Geometry check sheet. Reference: the model listing, model coordinates, mm. Face numbers are marked on the shaded views. Give positions to 0.01 mm unless a question says otherwise; leave off trailing zeros. Write each loop counter-clockwise with the first axis right and the second up, starting at its lowest first coordinate (ties: lowest second). Pieces come first, ordered by that corner, then holes. Notation, with made-up numbers: (82.5, 85) - (94.5, 85) arc R14 cw to (94.5, 93) - close; hole circle Ø10 at (3.5, 63). An arc over 180 degrees is marked (long way). One line per question, with ' | ' between items. Start each with the question number.
Q1. Gauge pin test, flat ends, axial feed: P1, Ø1, axis at x = 6, y = 3, coming from the -Z side; P2, Ø1.5, axis at y = 3, z = -3.5, coming from the -X side; P3, Ø5, axis at x = 60, z = 0, coming from the +Y side. Record the tip position at first contact, or that the pin passes through.
Q2. Thickness scan on L1, parallel to X at y = 2.55, z = -1.25; L2, parallel to X at y = 4.05, z = -1.5; L3, parallel to Z at x = -2.5, y = 4.15. Record the ranges inside material, lowest first. Write a range as [from, to].
Q3. Section check A-A on y = 2.7. Record the boundary of the cut face in (x, z), and give its area (3 significant figures).
Q4. Section check C-C on z = -9. Record the boundary of the cut face in (x, y), and give its area (3 significant figures).
Q5. Release check for a two-part mould opening along Z. For the marked faces 1, 2, 3 and 4 record: +Z half, -Z half, draft (parallel to the pull), parting line (faces both ways), or undercut.
Q6. Section check B-B on x = 31.5. Record the boundary of the cut face in (y, z).
```python
from build123d import *

# Parameters (mm, degrees)
SKETCH_1_R      = 12.5
SKETCH_1_R_2    = 8
SKETCH_1_R_3    = 3.05
EXTRUDE_1_DEPTH = 5


with BuildPart() as part:
    # 草图1 → 凸台-拉伸1 (new body)
    # profile 1 of 3: a face of its own
    with BuildSketch(Plane(origin=(0, 0, 0), x_dir=(1, 0, 0), z_dir=(0, 1, 0))):
        with BuildLine():
            ThreePointArc((12.5, 0), (9.164298937, -8.500919068), (0.9375, -12.464794172))
            Line((0.9375, -12.464794172), (60.6, -7.97746827))
            ThreePointArc((60.6, -7.97746827), (52, 0), (60.6, 7.97746827))
            Line((60.6, 7.97746827), (0.9375, 12.464794172))
            ThreePointArc((0.9375, 12.464794172), (9.164298937, 8.500919068), (12.5, 0))
        make_face()
    # profile 2 of 3: a face of its own
    with BuildSketch(Plane(origin=(0, 0, 0), x_dir=(1, 0, 0), z_dir=(0, 1, 0))):
        Circle(SKETCH_1_R)
        Polygon((0, -7.071067812), (7.071067812, 0), (0, 7.071067812), (-7.071067812, 0), align=None, mode=Mode.SUBTRACT)
    # profile 3 of 3: a face of its own
    with BuildSketch(Plane(origin=(0, 0, 0), x_dir=(1, 0, 0), z_dir=(0, 1, 0))):
        with Locations((60, 0)):
            Circle(SKETCH_1_R_2)
        with Locations(Location((60, 0, 0), (0, 0, 270))):
            Circle(SKETCH_1_R_3, mode=Mode.SUBTRACT)
    extrude(amount=EXTRUDE_1_DEPTH)


solid = part.part
```
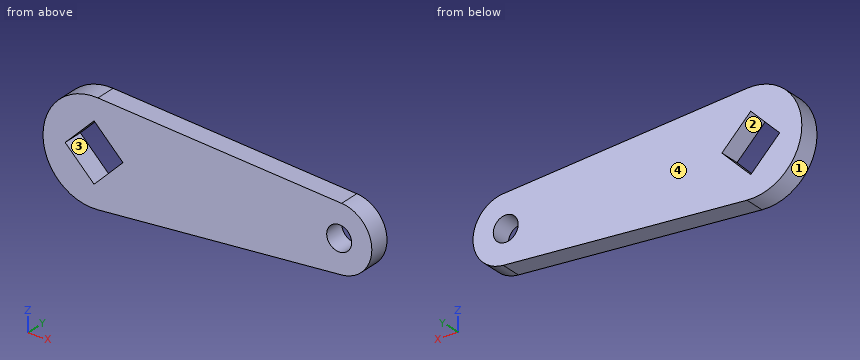
Working result:
1) P1: stops at z = -12.12 | P2: stops at x = -12.19 | P3: passes through
2) L1: x = [-12.44, -5.82], [5.82, 57.22], [62.78, 67.9] | L2: x = [-12.41, -5.57], [5.57, 57.34], [62.66, 67.86] | L3: z = [-12.25, -4.57], [4.57, 12.25]
3) outline: (0.94, -12.46) - (60.6, -7.98) arc R8 ccw to (60.6, 7.98) - (0.94, 12.46) arc R12.5 ccw (long way) to start; hole (-7.07, 0) - (0, -7.07) - (7.07, 0) - (0, 7.07) - close; hole circle Ø6.1 at (60, 0) | area: 1,450 mm2
4) outline: (-8.67, 0) - (47, 0) - (47, 5) - (-8.67, 5) - close | area: 278 mm2
5) face 1: parting line | face 2: undercut | face 3: undercut | face 4: draft
6) outline: (0, -10.17) - (5, -10.17) - (5, 10.17) - (0, 10.17) - close
